from build123d import *

# Parameters (mm, degrees)
ESBO_O1_W = 2.1
ESBO_O1_H = 30


with BuildPart() as part:
    # Sketch1 → Revolve1 (revolve)
    with BuildSketch(Plane.XY):
        with BuildLine():
            Line((0, -17.95), (0, -30))
            Line((0, -30), (10, -30))
            Line((10, -30), (12.679491924, -20))
            Line((12.679491924, -20), (22.320508076, -20))
            Line((22.320508076, -20), (25, -30))
            Line((25, -30), (35, -30))
            Line((35, -30), (35, -20))
            Line((35, -20), (44.5, -20))
            ThreePointArc((44.5, -20), (44.853553391, -19.853553391), (45, -19.5))
            Line((45, -19.5), (45, -7.95))
            Line((45, -7.95), (2.5, -7.95))
            Line((2.5, -7.95), (0, -17.95))
        make_face()
    revolve(axis=Axis((0, 0, 0), (1, 0, 0)))

    # Esboço1 → Broca de rosquear para tarraxa de M5x0.81 (revolve, cut)
    with BuildSketch(Plane.YZ.offset(40)):
        with Locations((1.05, 15)):
            Rectangle(ESBO_O1_W, ESBO_O1_H)
    revolve(axis=Axis((40, 0, -6.35), (0, 0, 1)), mode=Mode.SUBTRACT)


solid = part.part
Check sheet for the modelled part. Datum: model origin and axes. Units: mm. A direction names the side the tool comes from. Round coordinates to 2 decimals unless told otherwise and drop trailing zeros. Loops run counter-clockwise (first coordinate to the right, second up) from the corner with the lowest first, then second, coordinate; pieces in that order, holes last.
1. Set-up check for faces 5 (the cylindrical face through (39.816, 4.336, 19.524)), 6 (the cylindrical face through (5.07, 29.97, -1.32)), 7 (the cylindrical face through (17.567, 4.336, 19.524)): record each of +Z, -Z, +X, -X, +Y, -Y from which the full face is reachable in a straight line by a thin tool's end or side.
2. Sectioned sample at C-C on x = 32.5. Record the boundary of the cut face in (y, z).
3. Sectioned sample at D-D on x = 20.5. Record the boundary of the cut face in (y, z), and give its area (3 significant figures).
4. Sectioned sample at B-B on y = 0. Record the boundary of the cut face in (x, z), and give its area (3 significant figures).
5. Scan lines: probe 1 along Z at (x, y) = (18.5, 0); probe 2 along Z at (x, y) = (32, 0); probe 3 along X at (y, z) = (-22, -16.5). Record each from-to range of solid material in increasing order.
6. Mould release check, pull along Y, two halves, no side actions. Record for faces 1 (the flat face through (35, -6, 20)), 2 (the cylindrical face through (42.05, -0.46, 13.92)), 3 (the conical face through (22.5, -19.1, 7.9)), 4 (the cylindrical face through (23.45, 1.72, 7.76)): released by +Y, released by -Y, zero draft, split by the parting line, or undercut.
7. Sectioned sample at A-A on z = 0. Record the boundary of the cut face in (x, y), and give its area (3 significant figures).
8. Gauge pin test, flat ends, axial feed: pin 1 Ø5 at (y, z) = (24, -3.5) entering from +X; pin 2 Ø5 at (x, z) = (28, 20) entering from -Y; pin 3 Ø4 at (y, z) = (-8.5, 10) entering from -X. Record the tip position at first contact, or that the pin passes through.
Recorded:
1. face 5: +X
1. face 6: +X, -X
1. face 7: none
2. outline: circle Ø60 at (0, 0); hole circle Ø15.9 at (0, 0)
3. outline: circle Ø40 at (0, 0); hole circle Ø15.9 at (0, 0)
3. area: 1,060 mm2
4. outline: (0, -30) - (10, -30) - (12.68, -20) - (22.32, -20) - (25, -30) - (35, -30) - (35, -20) - (44.5, -20) arc R0.5 ccw to (45, -19.5) - (45, -7.95) - (2.5, -7.95) - (0, -17.95) - close; (0, 17.95) - (2.5, 7.95) - (37.9, 7.95) - (37.9, 20) - (35, 20) - (35, 30) - (25, 30) - (22.32, 20) - (12.68, 20) - (10, 30) - (0, 30) - close; (42.1, 7.95) - (45, 7.95) - (45, 19.5) arc R0.5 ccw to (44.5, 20) - (42.1, 20) - close
4. area: 1,460 mm2
5. probe 1: z = -20 to -7.95, 7.95 to 20
5. probe 2: z = -30 to -7.95, 7.95 to 30
5. probe 3: x = 0 to 10.67, 24.33 to 35
6. face 1: zero draft
6. face 2: undercut
6. face 3: split by the parting line
6. face 4: undercut
7. outline: (0, -30) - (10, -30) - (12.68, -20) - (22.32, -20) - (25, -30) - (35, -30) - (35, -20) - (44.5, -20) arc R0.5 ccw to (45, -19.5) - (45, -7.95) - (2.5, -7.95) - (0, -17.95) - close; (0, 17.95) - (2.5, 7.95) - (45, 7.95) - (45, 19.5) arc R0.5 ccw to (44.5, 20) - (35, 20) - (35, 30) - (25, 30) - (22.32, 20) - (12.68, 20) - (10, 30) - (0, 30) - close
7. area: 1,510 mm2
8. pin 1: stops at x = 35
8. pin 2: stops at y = -24.37
8. pin 3: stops at x = 0.71
